Geometry: see drawing. Coordinates: mm, zero at the bounding-box minimum. A direction names the side the tool comes from. Coordinates: 2 decimals unless noted, no trailing zeros. Write each loop counter-clockwise with the first axis right and the second up, starting at its lowest first coordinate (ties: lowest second). Pieces come first, ordered by that corner, then holes. Notation, with made-up numbers: (12, -16) -> (57, -16) arc R24 cw to (57, 17) -> close; hole circle Ø6 at (-22, -5). An arc over 180 degrees is marked (long way). Answer as a JSON object with one key per item and string values. Group by question number.
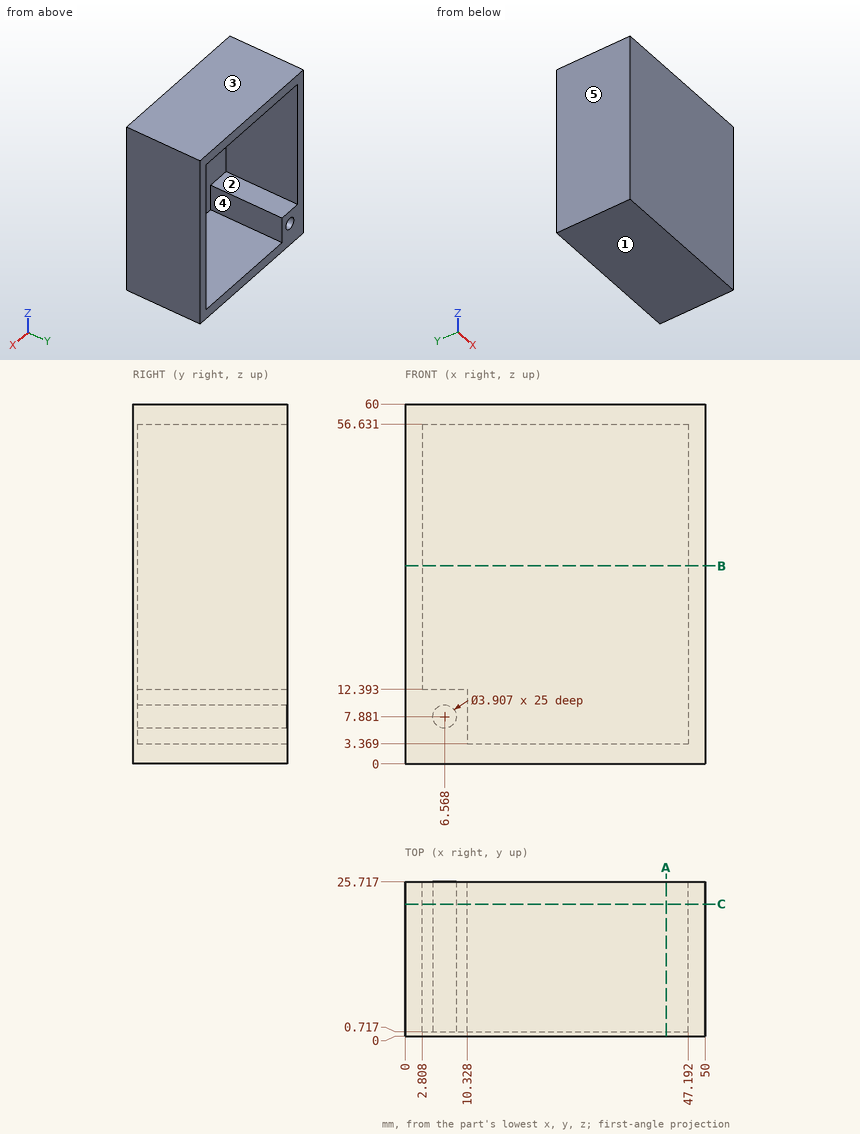
Item 1: Section C-C on y = 22. Output: boundary loops of the cut face in (x, z) (1 decimal).
Item 2: Mould query, pull axis X, two halves, no side actions, for the marked faces 3, 4 and 5. Classes: +X half, -X half, draft (parallel to the pull), parting line (faces both ways), or undercut.
Item 3: Section A-A on x = 43.5. Output: boundary loops of the cut face in (y, z).
Item 4: Set-up query: the marked faces 1 and 2. Return all of +Z, -Z, +X, -X, +Y, -Y with unobstructed straight access to the full face (end or side cutting, diameter ignored); none if empty.
Item 5: Contact query for a flat-ended pin moving along its axis: pin 1 (22 mm diameter, centred on x = 17, z = 30, fed in from +Y). Output: stop coordinate, or through.
Item 6: Section B-B on z = 33. Output: boundary loops of the cut face in (x, y).
Item 7: Ray query, L1, parallel to Z at x = 30, y = 19.75; L2, parallel to X at y = 22.25, z = 46.5; L3, parallel to X at y = 9.5, z = 10. Return the intervals inside material, ascending. Write a range as [from, to].
Answer sheet:
{
 "1": {"outline": "(0, 0) -> (50, 0) -> (50, 60) -> (0, 60) -> close; hole (2.8, 12.4) -> (10.3, 12.4) -> (10.3, 3.4) -> (47.2, 3.4) -> (47.2, 56.6) -> (2.8, 56.6) -> close; hole circle Ø3.9 at (6.6, 7.9)"},
 "2": {"face 3": "draft", "face 4": "undercut", "face 5": "-X half"},
 "3": {"outline": "(0, 0) -> (25.72, 0) -> (25.72, 3.37) -> (0.72, 3.37) -> (0.72, 56.63) -> (25.72, 56.63) -> (25.72, 60) -> (0, 60) -> close"},
 "4": {"face 1": "-Z, +X, -X, +Y, -Y", "face 2": "+Y"},
 "5": {"pin 1": "stops at y = 0.72"},
 "6": {"outline": "(0, 0) -> (50, 0) -> (50, 25.72) -> (47.19, 25.72) -> (47.19, 0.72) -> (2.81, 0.72) -> (2.81, 25.72) -> (0, 25.72) -> close"},
 "7": {"L1": "z = [0, 3.37], [56.63, 60]", "L2": "x = [0, 2.81], [47.19, 50]", "L3": "x = [0, 10.33], [47.19, 50]"}
}
